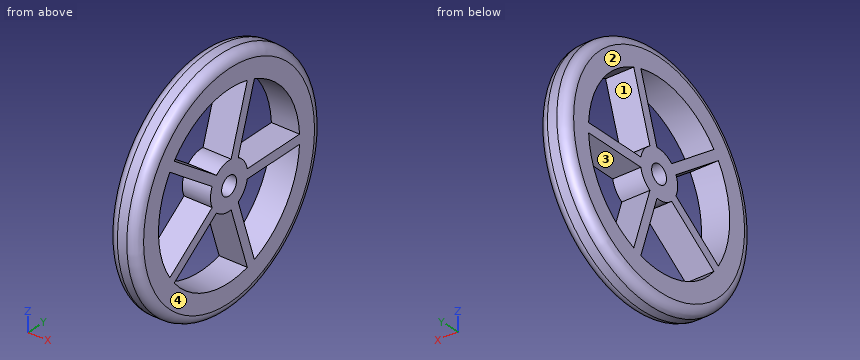
```python
from build123d import *

# Parameters (mm, degrees)
SKETCH1_R           = 250
SKETCH1_R_2         = 20
BOSS_EXTRUDE1_DEPTH = 60
FILLET1_R           = 20


with BuildPart() as part:
    # Sketch1 → Boss-Extrude1 (new body)
    with BuildSketch(Plane(origin=(0, 0, 0), x_dir=(0, 0, -1), z_dir=(1, 0, 0))):
        Circle(SKETCH1_R)
        Circle(SKETCH1_R_2, mode=Mode.SUBTRACT)
        with BuildLine():
            Line((183.540456446, 49.121287113), (49.682233573, 5.628113998))
            ThreePointArc((49.682233573, 5.628113998), (47.552825815, -15.450849719), (36.885648873, -33.755724066))
            Line((36.885648873, -33.755724066), (119.614580282, -147.622329558))
            ThreePointArc((119.614580282, -147.622329558), (180.700738096, -58.713228931), (183.540456446, 49.121287113))
        make_face(mode=Mode.SUBTRACT)
        with BuildLine():
            Line((-10, 189.73665961), (-10, 48.989794856))
            ThreePointArc((-10, 48.989794856), (-29.389262615, 40.450849719), (-43.501893686, 24.649244324))
            Line((-43.501893686, 24.649244324), (-177.360116559, 68.142417438))
            ThreePointArc((-177.360116559, 68.142417438), (-111.679197936, 153.713228931), (-10, 189.73665961))
        make_face(mode=Mode.SUBTRACT)
        with BuildLine():
            Line((10, 189.73665961), (10, 48.989794856))
            ThreePointArc((10, 48.989794856), (29.389262615, 40.450849719), (43.501893686, 24.649244324))
            Line((43.501893686, 24.649244324), (177.360116559, 68.142417438))
            ThreePointArc((177.360116559, 68.142417438), (111.679197936, 153.713228931), (10, 189.73665961))
        make_face(mode=Mode.SUBTRACT)
        with BuildLine():
            Line((103.434240394, -159.378034603), (20.705308985, -45.511429112))
            ThreePointArc((20.705308985, -45.511429112), (0, -50), (-20.705308985, -45.511429112))
            Line((-20.705308985, -45.511429112), (-103.434240394, -159.378034603))
            ThreePointArc((-103.434240394, -159.378034603), (0, -190), (103.434240394, -159.378034603))
        make_face(mode=Mode.SUBTRACT)
        with BuildLine():
            Line((-119.614580282, -147.622329558), (-36.885648873, -33.755724066))
            ThreePointArc((-36.885648873, -33.755724066), (-47.552825815, -15.450849719), (-49.682233573, 5.628113998))
            Line((-49.682233573, 5.628113998), (-183.540456446, 49.121287113))
            ThreePointArc((-183.540456446, 49.121287113), (-180.700738096, -58.713228931), (-119.614580282, -147.622329558))
        make_face(mode=Mode.SUBTRACT)
    extrude(amount=BOSS_EXTRUDE1_DEPTH)

    # Fillet1
    fillet1_edges = [part.edges().sort_by_distance(p)[0] for p in [
        (0, 0, 250),
        (60, 0, 250),
    ]]
    fillet(fillet1_edges, radius=FILLET1_R)


solid = part.part
```
For this review, take the finished solid that the model builds, in its own axes (mm). Face numbers are marked on the shaded views. A direction names the side the tool comes from. Coordinates: 2 decimals unless noted, no trailing zeros. Loops run counter-clockwise (first coordinate to the right, second up) from the corner with the lowest first, then second, coordinate; pieces in that order, holes last.
1. Insertion check: P1, Ø6, axis at y = -104.5, z = 183, coming from the -X side; P2, Ø1, axis at x = 49.5, z = 121.5, coming from the +Y side; P3, Ø8, axis at x = 53, y = 73, coming from the -Z side; P4, Ø1.5, axis at x = 14, y = 6.5, coming from the +Z side. Each pin has a flat end and moves straight along its axis. Give the tip position at first contact, or say it passes through.
2. Add section A-A, the plane z = 0. Give the boundary of the cut face in (x, y), then the cut area to 3 significant figures.
3. Add section C-C, the plane y = -9. Count the separate pieces of the cut face and the enclosed holes in it, then the cut area to 3 significant figures.
4. For line 1 (Y direction, x = 36, z = 0); line 2 (Y direction, x = 35.5, z = -39.5); line 3 (Y direction, x = 10, z = 138.5), list the stretches that pass through material, from the lowest coordinate up.
5. Mouldability with a two-part tool opening along Z and no side actions: class the marked faces 3 and 4 as +Z half, -Z half, draft (parallel to the pull), parting line (faces both ways), or undercut.
6. Add section B-B, the plane x = 31. Give the boundary of the cut face in (y, z).
7. For the marked faces 1 and 2, list the 3-axis set-ups (+Z, -Z, +X, -X, +Y, -Y) from which the entire face can be reached by the end or side of a thin tool; tool diameter is ignored.
Result:
1. P1: stops at x = 0
1. P2: stops at y = 216.15
1. P3: stops at z = -237.18
1. P4: stops at z = 249.21
2. outline: (0, -230) arc R20 ccw to (20, -250) - (40, -250) arc R20 ccw to (60, -230) - (60, -190) - (0, -190) - close; (0, -50) - (60, -50) - (60, -20) - (0, -20) - close; (0, 20) - (60, 20) - (60, 230) arc R20 ccw to (40, 250) - (20, 250) arc R20 ccw to (0, 230) - close
2. area: 18,900 mm2
3. separate pieces: 4
3. enclosed holes: 0
3. area: 10,600 mm2
4. line 1: y = -250 to -190, -50 to -20, 20 to 250
4. line 2: y = -246.86 to -185.85, -71.38 to -37.35, -30.66 to 30.66, 185.85 to 246.86
4. line 3: y = -204.9 to -130.07, 34.49 to 55.52, 130.07 to 204.9
5. face 3: undercut
5. face 4: draft
6. outline: circle Ø500 at (0, 0); hole (-159.38, -103.43) - (-45.51, -20.71) arc R50 cw to (-45.51, 20.71) - (-159.38, 103.43) arc R190 ccw to start; hole (-147.62, -119.61) arc R190 ccw to (49.12, -183.54) - (5.63, -49.68) arc R50 cw to (-33.76, -36.89) - close; hole (-147.62, 119.61) - (-33.76, 36.89) arc R50 cw to (5.63, 49.68) - (49.12, 183.54) arc R190 ccw to start; hole circle Ø40 at (0, 0); hole (24.65, -43.5) - (68.14, -177.36) arc R190 ccw to (189.74, -10) - (48.99, -10) arc R50 cw to start; hole (24.65, 43.5) arc R50 cw to (48.99, 10) - (189.74, 10) arc R190 ccw to (68.14, 177.36) - close
7. face 1: +X, -X
7. face 2: +Z, -Z, -X, +Y, -Y
